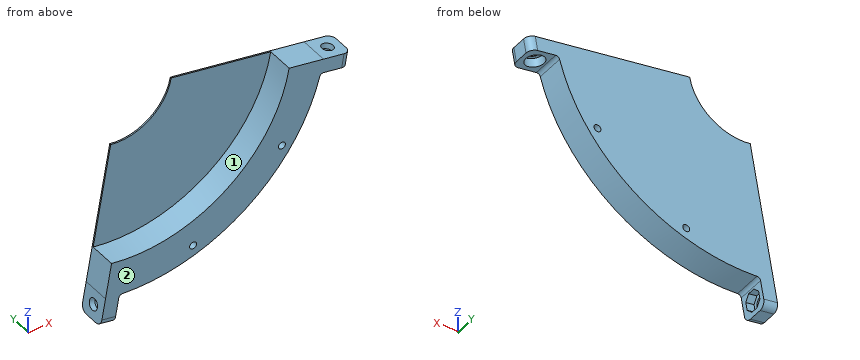
Autodesk Inventor part; units mm, degrees
ref_plane "YZ Plane" through (0, 0, 0) normal (1, 0, 0) x (0, 1, 0)
ref_plane "XZ Plane" through (0, 0, 0) normal (0, 1, 0) x (-1, 0, 0)
ref_plane "XY Plane" through (0, 0, 0) normal (0, 0, 1) x (1, 0, 0)
sketch "Sketch1" plane through (0, 0, 0) normal (0, 1, 0) x (-1, 0, 0)
  circle A0 centre (0, 0) radius 135
  circle A1 centre (0, 0) radius 110
  dimension "d0" = 270
  dimension "d1" = 220
extrude "Extrusion1" add sketch "Sketch1" along normal mid plane 20
sketch "Sketch2" plane through (0, 10, 0) normal (0, 1, 0) x (1, 0, 0)
  circle A0 centre (0, 0) radius 37.5
  circle A1 centre (0, 0) radius 135
  dimension "d4" = 75
  dimension "d20" = 270
extrude "Extrusion2" add sketch "Sketch2" against normal blind 1
sketch "Sketch3" plane through (0, 10, 0) normal (0, 1, 0) x (1, 0, 0)
  circle A0 centre (0, 0) radius 127.5
  circle A1 centre (127.5, 0) radius 2.5
  circle A2 centre (103.1497, 74.9426) radius 2.5
  circle A3 centre (39.3997, 121.2597) radius 2.5
  circle A4 centre (-39.3997, 121.2597) radius 2.5
  circle A5 centre (-103.1497, 74.9426) radius 2.5
  circle A6 centre (-127.5, 0) radius 2.5
  circle A7 centre (-103.1497, -74.9426) radius 2.5
  circle A8 centre (-39.3997, -121.2597) radius 2.5
  circle A9 centre (39.3997, -121.2597) radius 2.5
  circle A10 centre (103.1497, -74.9426) radius 2.5
  dimension "d7" = 255
  dimension "d8" = 5
  dimension "d11" = 360
hole "Hole1" at (127.5, 10, 0) at (103.1497, 10, 74.9426) at (39.3997, 10, 121.2597) at (-39.3997, 10, 121.2597) at (-103.1497, 10, 74.9426) at (-127.5, 10, 0) at (-103.1497, 10, -74.9426) at (-39.3997, 10, -121.2597) at (39.3997, 10, -121.2597) at (103.1497, 10, -74.9426) direction (0, -1, 0) diameter 5 end through all
sketch "Sketch4" plane through (0, -10, 0) normal (0, -1, 0) x (1, 0, 0)
  circle A0 centre (0, 0) radius 135
  line L0 (0, 0) -> (132.949, -23.4425)
  line L1 (0, 0) -> (135, 0) construction
  line L2 (0, 0) -> (-23.4425, -132.949)
  circle A1 centre (0, 0) radius 135
  line L3 (0, 0) -> (135, 0) construction
  line L4 (0, 0) -> (-132.949, 23.4425)
  dimension "d21" = 135
  dimension "d22" = 10
  dimension "d23" = 100
extrude "Extrusion3" cut sketch "Sketch4" against normal through all contours A0 L0 L4 | L4 L2 A0
sketch "Sketch5" plane through (-23.4425, -10, -132.949) normal (-0.9848, 0, 0.1736) x (0.1736, 0, 0.9848)
  line L0 (135, 20) -> (0, 20)
  line L1 (2.5, 20) -> (-15, 20)
  line L2 (-20, 15) -> (-20, 5)
  line L3 (-15, 0) -> (2.5, 0)
  line L4 (2.5, 0) -> (2.5, 20)
  line L5 (0, 0) -> (0, 20)
  arc A0 (-20, 5) -> (-15, 0) centre (-15, 5) ccw
  arc A1 (-15, 20) -> (-20, 15) centre (-15, 15) ccw
  point P0 (135, 10)
  point P1 (-20, 0)
  point P2 (-20, 20)
  point P3 (0, 20)
  dimension "d26" = 22.5
  dimension "d27" = 20
  dimension "d28" = 20
  dimension "d29" = 5
extrude "Extrusion4" add sketch "Sketch5" against normal blind 10
fillet "Fillet1" radius 2.5 1 edges at (-13.53, 0, -134.3203)
sketch "Sketch6" plane through (132.949, -10, -23.4425) normal (0.1736, 0, 0.9848) x (0.9848, 0, -0.1736)
  line L0 (-122.7273, 0) -> (0, 0)
  line L1 (-2.5, 0) -> (15, 0)
  line L2 (20, 5) -> (20, 15)
  line L3 (15, 20) -> (-2.5, 20)
  line L4 (-2.5, 20) -> (-2.5, 0)
  line L5 (0, 20) -> (0, 0)
  arc A0 (20, 15) -> (15, 20) centre (15, 15) ccw
  arc A1 (15, 0) -> (20, 5) centre (15, 5) ccw
  point P0 (-135, 10)
  point P1 (20, 20)
  point P2 (20, 0)
  point P3 (0, 0)
  dimension "d33" = 22.5
  dimension "d34" = 20
  dimension "d35" = 20
  dimension "d36" = 5
extrude "Extrusion5" add sketch "Sketch6" against normal blind 10
fillet "Fillet2" radius 2.5 1 edges at (130.8473, 0, -33.2262)
sketch "Sketch7" plane through (-13.5944, -10, -134.6855) normal (0.9848, 0, -0.1736) x (-0.1736, 0, -0.9848)
  line L0 (16.6, 12.7338) -> (16.6, 7.2662)
  line L1 (16.6, 7.2662) -> (12.7338, 3.4)
  line L2 (12.7338, 3.4) -> (7.2662, 3.4)
  line L3 (7.2662, 3.4) -> (3.4, 7.2662)
  line L4 (3.4, 7.2662) -> (3.4, 12.7338)
  line L5 (3.4, 12.7338) -> (7.2662, 16.6)
  line L6 (7.2662, 16.6) -> (12.7338, 16.6)
  line L7 (12.7338, 16.6) -> (16.6, 12.7338)
  line L8 (20, 5) -> (20, 15)
  line L9 (1.9306, 0) -> (15, 0)
  point P0 (-135, 10)
  point P1 (10, 10)
  point P2 (20, 10)
  dimension "d40" = 10
  dimension "d41" = 10
  dimension "d42" = 13.2
extrude "Extrusion6" cut sketch "Sketch7" against normal blind 6
sketch "Sketch8" plane through (-19.5033, -10, -133.6436) normal (0.9848, 0, -0.1736) x (-0.1736, 0, -0.9848)
  line L0 (1.9306, 0) -> (15, 0)
  line L1 (20, 5) -> (20, 15)
  point P0 (-135, 10)
  point P1 (10, 10)
  dimension "d45" = 10
  dimension "d46" = 10
hole "Hole2" at (-21.2398, 0, -143.4917) direction (-0.9848, 0, 0.1736) diameter 8.2 end through all
sketch "Sketch9" plane through (131.2126, -10, -33.2906) normal (-0.1736, 0, -0.9848) x (-0.9848, 0, 0.1736)
  line L0 (-20, 15) -> (-20, 5)
  line L1 (-1.9306, 20) -> (-15, 20)
  point P0 (135, 10)
  point P1 (-10, 10)
  dimension "d54" = 10
  dimension "d55" = 10
hole "Hole3" at (141.0606, 0, -35.0271) direction (0.1736, 0, 0.9848) diameter 8.2 end through all counterbore diameter 13.2 counterbore depth 6
properties part number "Cylinder Spacer 25mm_Q2+4"
Can you work these out from the model? Positions are in its coordinate system, mm. Face numbers are marked on the shaded views. Give positions to 0.01 mm unless a question says otherwise; leave off trailing zeros. Loops run counter-clockwise (first coordinate to the right, second up) from the corner with the lowest first, then second, coordinate; pieces in that order, holes last. Notation, with made-up numbers: M -31.5,65 L -0.5,65 A10 cw -0.5,77 Z; hole C 1.25,45.5 d7. An arc over 180 degrees is marked long. Use CSV: the item, a comma, the result in double quotes. Start each with the question number.
1. If I drill on L1, parallel to Y at x = 27, z = -87.5; L2, parallel to Z at x = 39, y = 2.75; L3, parallel to Z at x = 41, y = -2, over which ranges is the centre line in solid material (lowest first)?
2. Imagine slicing it at A-A, the plane z = -82.5. Write out the boundary of the cut face in (x, y).
3. If we mould it in two halves opening along X, with no side actions, what happens to the marked faces 1 and 2? For each: released by +X, released by -X, zero draft, split by the parting line, or undercut.
4. Imagine slicing it at B-B, the plane x = 67. Write out the boundary of the cut face in (y, z).
5. For P1, Ø2, axis at x = 120.5, y = 6.5, coming from the -Z side; P2, Ø2, axis at x = 110.5, y = 4.5, coming from the +Z side; P3, Ø8, axis at y = -3.5, z = -128.5, coming from the -X side, each with a flat end and sliding along its axis, tell me the tip position at first contact or that it passes through.
6. Imagine slicing it at D-D, the plane z = -16.5. Write out the boundary of the cut face in (x, y), plus the area to 3 significant figures.
7. Imagine slicing it at C-C, the plane x = 126.5. Write out the boundary of the cut face in (y, z), plus the area to 3 significant figures.
Response values:
1,L1,"9 to 10"
1,L2,"-129.24 to -123.73, -118.79 to -102.85"
1,L3,"-128.62 to -123.18, -119.34 to -102.07"
2,outline,"M -14.55,9 L 72.76,9 L 72.76,-10 L 106.86,-10 L 106.86,10 L -14.55,10 Z"
3,face 1,"undercut"
3,face 2,"zero draft"
4,outline,"M -10,-117.2 L 10,-117.2 L 10,-11.81 L 9,-11.81 L 9,-87.24 L -10,-87.24 Z"
5,P1,"z = -62.81"
5,P2,"z = -19.31"
5,P3,"x = -23.36"
6,outline,"M 33.67,9 L 93.58,9 L 93.58,10 L 33.67,10 Z"
6,area,"59.9 mm^2"
7,outline,"M -10,-47.15 L 10,-47.15 L 10,-22.31 L -10,-22.31 Z"
7,area,"497 mm^2"
